```python
from build123d import *

# Parameters (mm, degrees)
SKETCH_1_W          = 70
SKETCH_1_H          = 10
EXTRUDE_1_DEPTH     = 20
SKETCH_2_R          = 1.7
CUT_EXTRUDE_1_DEPTH = 20
SKETCH_3_W          = 30
SKETCH_3_H          = 1
CUT_EXTRUDE_2_DEPTH = 10
FILLET_1_R          = 5
FILLET_2_R          = 3
FILLET_3_R          = 1


with BuildPart() as part:
    # 草图1 → 凸台-拉伸1 (new body)
    with BuildSketch(Plane(origin=(0, 0, 0), x_dir=(1, 0, 0), z_dir=(0, 1, 0))):
        Rectangle(SKETCH_1_W, SKETCH_1_H)
    extrude(amount=EXTRUDE_1_DEPTH)

    # 草图2 → 切除-拉伸1 (cut)
    with BuildSketch(Plane(origin=(0, 20, 0), x_dir=(1, 0, 0), z_dir=(0, 1, 0))):
        with Locations(Location((-30, 0, 0), (0, 0, 270))):
            Circle(SKETCH_2_R)
        with Locations(Location((30, 0, 0), (0, 0, 90))):
            Circle(SKETCH_2_R)
    extrude(amount=-CUT_EXTRUDE_1_DEPTH, mode=Mode.SUBTRACT)

    # 草图3 → 切除-拉伸2 (cut)
    with BuildSketch(Plane.XY.offset(5)):
        Polygon((-25, 0), (25, 0), (25, 6), (19, 12), (-19, 12), (-25, 6), align=None)
        with Locations((0, 19.5)):
            Rectangle(SKETCH_3_W, SKETCH_3_H)
    extrude(amount=-CUT_EXTRUDE_2_DEPTH, mode=Mode.SUBTRACT)

    # 圆角1
    fillet_1_edges = [part.edges().sort_by_distance(p)[0] for p in [
        (-25, 6, 0),
        (-19, 12, 0),
        (19, 12, 0),
        (25, 6, 0),
    ]]
    fillet(fillet_1_edges, radius=FILLET_1_R)

    # 圆角2
    fillet_2_edges = [part.edges().sort_by_distance(p)[0] for p in [
        (35, 10, 5),
        (-35, 10, 5),
        (-35, 10, -5),
        (35, 10, -5),
    ]]
    fillet(fillet_2_edges, radius=FILLET_2_R)

    # 圆角3
    fillet_3_edges = [part.edges().sort_by_distance(p)[0] for p in [
        (15, 19, 0),
        (-15, 19, 0),
    ]]
    fillet(fillet_3_edges, radius=FILLET_3_R - 0.0001)  # a hair under: the kernel refuses the full size


solid = part.part
```
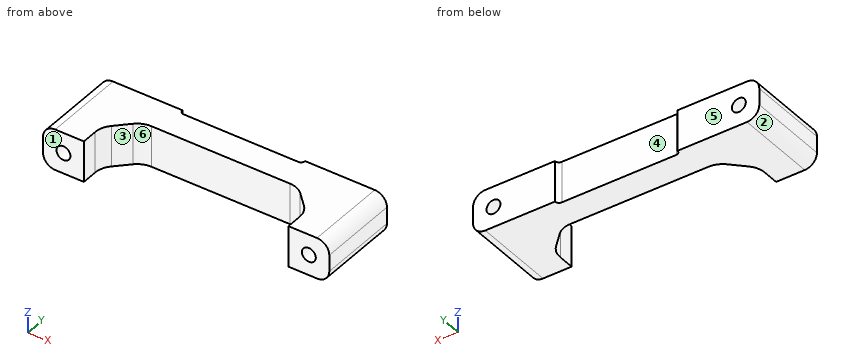
Geometry check sheet. Reference: the model listing, model coordinates, mm. Face numbers are marked on the shaded views. A direction names the side the tool comes from. Coordinates: 2 decimals unless noted, no trailing zeros. Order: outer loops, then holes, each group sorted by start corner. A loop starts at its lowest first (then second) coordinate and runs counter-clockwise, first axis right, second up. Notation, with made-up numbers: M 78.5,37 L 132.5,37 A29 cw 132.5,68 Z; hole C 44,23.25 d11. An arc over 180 degrees is marked long. Answer as a JSON object with one key per item and string values.
Q1. Release check for a two-part mould opening along X. For the marked faces 1, 2 and 3 record: released by +X, released by -X, zero draft, split by the parting line, or undercut.
Results are:
{"face 1": "zero draft", "face 2": "released by -X", "face 3": "undercut"}
Q2. Cross-section at C-C on y = 17.5. Record the cut outline in (x, z).
Results are:
{"outline": "M -35,-2 A3 ccw -32,-5 L 32,-5 A3 ccw 35,-2 L 35,2 A3 ccw 32,5 L -32,5 A3 ccw -35,2 Z; hole C -30,0 d3.4; hole C 30,0 d3.4"}
Q3. Tool access check on the marked faces 4, 5 and 6. Record the directions out of +Z, -Z, +X, -X, +Y, -Y that give a thin tool (end or side, any length) a straight path to the whole face; none if there is none.
Results are:
{"face 4": "+Z, -Z, +Y", "face 5": "+Z, -Z, +X, -X, +Y", "face 6": "+Z, -Z, -Y"}
Q4. Cross-section at A-A on y = 9.25. Record the cut outline in (x, z), and give its area (3 significant figures).
Results are:
{"outline": "M -35,-2 A3 ccw -32,-5 L -21.75,-5 L -21.75,5 L -32,5 A3 ccw -35,2 Z; M 21.75,-5 L 32,-5 A3 ccw 35,-2 L 35,2 A3 ccw 32,5 L 21.75,5 Z; hole C -30,0 d3.4; hole C 30,0 d3.4", "area": "239 mm²"}
Q5. Depth check by flat-ended pin: pin 1 Ø2 at (x, z) = (30, 0) entering from +Y; pin 2 Ø3 at (x, z) = (0.5, 0) entering from -Y; pin 3 Ø5 at (x, z) = (-0.5, -1) entering from +Y. Enter the tip coordinate at first touch or a pass-through.
Results are:
{"pin 1": "passes through", "pin 2": "stops at y = 12", "pin 3": "stops at y = 19"}
Q6. Scan lines: line 1 (X direction, y = 14.25, z = 0); line 2 (Z direction, x = 30, y = 14); line 3 (X direction, y = 8, z = 0). Record each from-to range of solid material in increasing order.
Results are:
{"line 1": "x = -35 to -31.7, -28.3 to 28.3, 31.7 to 35", "line 2": "z = -5 to -1.7, 1.7 to 5", "line 3": "x = -35 to -31.7, -28.3 to -23, 23 to 28.3, 31.7 to 35"}
Q7. Cross-section at B-B on x = 30. Record the cut outline in (y, z), and give its area (3 significant figures).
Results are:
{"outline": "M 0,-5 L 20,-5 L 20,-1.7 L 0,-1.7 Z; M 0,1.7 L 20,1.7 L 20,5 L 0,5 Z", "area": "132 mm²"}
